Geometry: final body of the model. Coordinates: model frame, mm. A direction names the side the tool comes from. Coordinates: 2 decimals unless noted, no trailing zeros. Write each loop counter-clockwise with the first axis right and the second up, starting at its lowest first coordinate (ties: lowest second). Pieces come first, ordered by that corner, then holes.
from build123d import *

# Parameters (mm, degrees)
F1_DEPTH = 10


with BuildPart() as f1:
    # F0 (on Top) → F1 (new body)
    with BuildSketch(Plane.XY):
        with BuildLine():
            ThreePointArc((-9.6618913839, 6.0816285435), (-10.2767491333, 8.754632337), (-7.5396319115, 8.9312354108))
            Line((-7.5396319115, 8.9312354108), (-4.9405973193, 6.2455355452))
            Line((-4.9405973193, 6.2455355452), (-2.8629372828, 3.9173089899))
            ThreePointArc((-2.8629372828, 3.9173089899), (-1.2204668488, 3.1932707933), (-1.9445042126, 4.8357415944))
            Line((-1.9445042126, 4.8357415944), (-4.5220414177, 7.7984281816))
            Line((-4.5220414177, 7.7984281816), (-6.8499312622, 10.3170876293))
            ThreePointArc((-6.8499312622, 10.3170876293), (-11.4164551285, 9.7328706229), (-10.9552195609, 5.1522908034))
            add(Edge.make_bspline(
                [(-10.9552195609, 5.1522908034), (-10.6926542112, 4.9714270901), (-10.058152243, 4.5343611094), (-8.8142262778, 4.1882031461), (-8.0850534141, 3.9852899499)],
                knots=[0, 0, 0, 0, 0.4138132943, 1, 1, 1, 1], degree=3))
            ThreePointArc((-8.0850534141, 3.9852899499), (-6.0877209286, -1.2198178636), (-11.662869985, -1.2057677011))
            Line((-11.662869985, -1.2057677011), (-12.6730389893, -0.1474826422))
            ThreePointArc((-12.6730389893, -0.1474826422), (-13.8998387132, 0.3415873294), (-13.6815843859, -0.9609456062))
            Line((-13.6815843859, -0.9609456062), (-12.9269978385, -2.067672831))
            ThreePointArc((-12.9269978385, -2.067672831), (-4.8279533498, -2.0880835662), (-7.7294873707, 5.4734003194))
            Line((-7.7294873707, 5.4734003194), (-9.6618913839, 6.0816285435))
        make_face()
    extrude(amount=F1_DEPTH)


solid = f1.part
Item 1: Section A-A, the plane y = 8.5. Output: boundary loops of the cut face in (x, z), plus the area to 3 significant figures.
Derived:
outline: (-12.03, 0) - (-10.44, 0) - (-10.44, 10) - (-12.03, 10) - close; (-7.12, 0) - (-5.17, 0) - (-5.17, 10) - (-7.12, 10) - close
area: 35.5 mm2
Item 2: Set-up query: faces 5 (the flat face through (-6.26, 7.61, 4.93)), 6 (the flat face through (-13.31, -1.507, 4.93)). Return all of +Z, -Z, +X, -X, +Y, -Y with unobstructed straight access to the full face (end or side cutting, diameter ignored); none if empty.
Derived:
face 5: +Z, -Z
face 6: +Z, -Z, -X, -Y
Item 3: Material intervals for probe 1 along Y at (x, z) = (-6, 1.25) (1 decimal); probe 2 along Y at (x, z) = (-6.25, 8.25); probe 3 along X at (y, z) = (0.75, 1.25), sorted ascending.
Derived:
probe 1: y = -3.3 to -1.1, 2.5 to 4.7, 7.3 to 9.4
probe 2: y = -3.45 to -1.44, 2.83 to 4.85, 7.6 to 9.67
probe 3: x = -5.49 to -3.96
Item 4: Section B-B, the plane y = -0.5. Output: boundary loops of the cut face in (x, z), plus the area to 3 significant figures.
Derived:
outline: (-14.14, 0) - (-12.34, 0) - (-12.34, 10) - (-14.14, 10) - close; (-5.71, 0) - (-4.11, 0) - (-4.11, 10) - (-5.71, 10) - close
area: 34.0 mm2
Item 5: Pull-direction query (X, two-part tool) for faces 1 (the cylindrical face through (-11.37, 9.79, 4.93)), 2 (the flat face through (-7, 4, 10)), 3 (the flat face through (-8.682, 5.773, 4.93)), 4 (the flat face through (-3.22, 6.3, 4.93)); classes: released by +X, released by -X, zero draft, split by the parting line, or undercut.
Derived:
face 1: split by the parting line
face 2: zero draft
face 3: undercut
face 4: released by +X
Item 6: Pin query (flat end, axial travel): pin 1 (1 mm diameter, centred on x = -10, z = 4, fed in from +Y); pin 2 (3 mm diameter, centred on y = 7.5, z = 2, fed in from -X). Return the tip coordinate at first contact, or that it passes through.
Derived:
pin 1: stops at y = 10.91
pin 2: stops at x = -12.13
Item 7: Section C-C, the plane x = -8.5. State how many separate pieces and enclosed holes the cut face has, plus the area to 3 significant figures.
Derived:
separate pieces: 3
enclosed holes: 0
area: 46.7 mm2
Item 8: Section D-D, the plane y = 2.5. Output: boundary loops of the cut face in (x, z).
Derived:
outline: (-6.01, 0) - (-4.3, 0) - (-4.3, 10) - (-6.01, 10) - close
